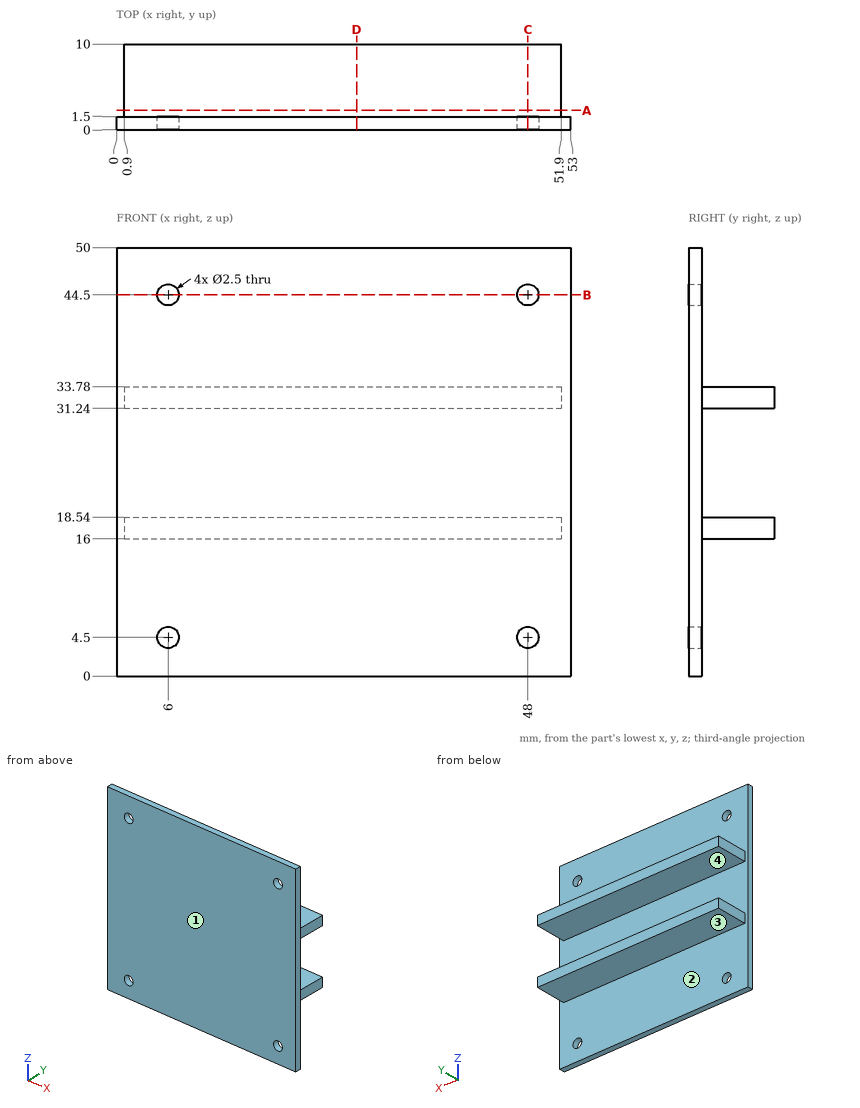
Geometry: see drawing. Coordinates: mm, zero at the bounding-box minimum. Give positions to 0.01 mm unless a question says otherwise; leave off trailing zeros. Loops run counter-clockwise (first coordinate to the right, second up) from the corner with the lowest first, then second, coordinate; pieces in that order, holes last. Notation, with made-up numbers: (6.25, 65.25) -> (56.25, 65.25) arc R6 cw to (56.25, 69.25) -> close; hole circle Ø1 at (10.5, 86.5). An arc over 180 degrees is marked (long way). Answer as a JSON object with one key per item and string values. Group by question number.
Item 1: Cut plane C-C, the plane x = 48. Return the cut outline in (y, z).
Item 2: Pull-direction query (Z, two-part tool) for the marked faces 1, 2, 3 and 4; classes: released by +Z, released by -Z, zero draft, split by the parting line, or undercut.
Item 3: Pin query (flat end, axial travel): P1, Ø3, axis at x = 20, y = 4, coming from the +Z side; P2, Ø2, axis at x = 43, z = 11.5, coming from the +Y side; P3, Ø6, axis at y = 1.5, z = 40.5, coming from the -X side; P4, Ø1.3, axis at y = 5.5, z = 33, coming from the -X side. Return the tip coordinate at first contact, or that it passes through.
Item 4: Cut plane D-D, the plane x = 28. Return the cut outline in (y, z), and give its area (3 significant figures).
Item 5: Cut plane B-B, the plane z = 44.5. Return the cut outline in (x, y).
Item 6: Cut plane A-A, the plane y = 2.25. Return the cut outline in (x, z), and give its area (3 significant figures).
Item 7: Line query: probe 1 along Z at (x, y) = (6, 0.75); probe 2 along X at (y, z) = (0.8, 4.5); probe 3 along Z at (x, y) = (25, 7.5). Output: solid intervals per line, ascending.
Checks:
{
 "1": {"outline": "(0, 0) -> (1.5, 0) -> (1.5, 3.25) -> (0, 3.25) -> close; (0, 5.75) -> (1.5, 5.75) -> (1.5, 16) -> (10, 16) -> (10, 18.54) -> (1.5, 18.54) -> (1.5, 31.24) -> (10, 31.24) -> (10, 33.78) -> (1.5, 33.78) -> (1.5, 43.25) -> (0, 43.25) -> close; (0, 45.75) -> (1.5, 45.75) -> (1.5, 50) -> (0, 50) -> close"},
 "2": {"face 1": "zero draft", "face 2": "undercut", "face 3": "released by -Z", "face 4": "undercut"},
 "3": {"P1": "stops at z = 33.78", "P2": "stops at y = 1.5", "P3": "stops at x = 0", "P4": "stops at x = 0.9"},
 "4": {"outline": "(0, 0) -> (1.5, 0) -> (1.5, 16) -> (10, 16) -> (10, 18.54) -> (1.5, 18.54) -> (1.5, 31.24) -> (10, 31.24) -> (10, 33.78) -> (1.5, 33.78) -> (1.5, 50) -> (0, 50) -> close", "area": "118 mm²"},
 "5": {"outline": "(0, 0) -> (4.75, 0) -> (4.75, 1.5) -> (0, 1.5) -> close; (7.25, 0) -> (46.75, 0) -> (46.75, 1.5) -> (7.25, 1.5) -> close; (49.25, 0) -> (53, 0) -> (53, 1.5) -> (49.25, 1.5) -> close"},
 "6": {"outline": "(0.9, 16) -> (51.9, 16) -> (51.9, 18.54) -> (0.9, 18.54) -> close; (0.9, 31.24) -> (51.9, 31.24) -> (51.9, 33.78) -> (0.9, 33.78) -> close", "area": "259 mm²"},
 "7": {"probe 1": "z = 0 to 3.25, 5.75 to 43.25, 45.75 to 50", "probe 2": "x = 0 to 4.75, 7.25 to 46.75, 49.25 to 53", "probe 3": "z = 16 to 18.54, 31.24 to 33.78"}
}
